from build123d import *

# Parameters (mm, degrees)
SKETCH_1_W          = 30
SKETCH_1_H          = 13
EXTRUDE_1_DEPTH     = 10
SKETCH_2_W          = 24
SKETCH_2_H          = 10
CUT_EXTRUDE_1_DEPTH = 20
SKETCH_3_R          = 3
EXTRUDE_2_DEPTH     = 5
SKETCH_4_R          = 3
CUT_EXTRUDE_2_DEPTH = 39.288379438
FILLET_1_R          = 6


with BuildPart() as part:
    # 草图1 → 凸台-拉伸1 (new, symmetric)
    with BuildSketch(Plane(origin=(0, 0, 0), x_dir=(1, 0, 0), z_dir=(0, 1, 0))):
        Rectangle(SKETCH_1_W, SKETCH_1_H)
    extrude(amount=EXTRUDE_1_DEPTH, both=True)

    # 草图2 → 切除-拉伸1 (cut)
    with BuildSketch(Plane(origin=(0, 0, -6.5), x_dir=(-1, 0, 0), z_dir=(0, 0, -1))):
        with Locations((15, 0)):
            Rectangle(SKETCH_2_W, SKETCH_2_H)
    extrude(amount=-CUT_EXTRUDE_1_DEPTH, mode=Mode.SUBTRACT)

    # 草图3 → 凸台-拉伸2 (add)
    with BuildSketch(Plane(origin=(0, 10, 0), x_dir=(1, 0, 0), z_dir=(0, 1, 0))):
        with BuildLine():
            Line((-3.690899012, 26.00908083), (-15, 6.5))
            Line((-15, 6.5), (-1, 6.5))
            Line((-1, 6.5), (6.712455076, 20.028415898))
            ThreePointArc((6.712455076, 20.028415898), (4.49035189, 28.201710831), (-3.690899012, 26.00908083))
        make_face()
        with Locations(Location((1.5, 23, 0), (0, 0, 270))):
            Circle(SKETCH_3_R, mode=Mode.SUBTRACT)
    extrude(amount=-EXTRUDE_2_DEPTH)

    # 草图4 → 切除-拉伸2 (cut, through all)
    with BuildSketch(Plane(origin=(0, 10, 0), x_dir=(1, 0, 0), z_dir=(0, 1, 0))):
        with Locations(Location((-9, 0, 0), (0, 0, 270))):
            Circle(SKETCH_4_R)
    extrude(amount=-CUT_EXTRUDE_2_DEPTH, mode=Mode.SUBTRACT)

    # 圆角1
    fillet_1_edges = [part.edges().sort_by_distance(p)[0] for p in [
        (-15, -7.5, 6.5),
        (-15, -7.5, -6.5),
        (-15, 7.5, 6.5),
    ]]
    fillet(fillet_1_edges, radius=FILLET_1_R)


solid = part.part
Geometry: final body of the model. Coordinates: model frame, mm. A direction names the side the tool comes from. Coordinates: 2 decimals unless noted, no trailing zeros. Order: outer loops, then holes, each group sorted by start corner. A loop starts at its lowest first (then second) coordinate and runs counter-clockwise, first axis right, second up.
(1) Draft query along Y for faces 5 (the face through (-9.266, 7.535, -16.391)), 6 (the face through (-4, 10, -8)), 7 (the face through (-6, -5, -2)), 8 (the face through (-3, 0, 0)). Return one class per face: pulls with the +Y half, pulls with the -Y half, needs draft (parallel to the pull), parting line crosses it, or undercut.
(2) Section query D-D (y = -8.5). Return the cut outline in (x, z).
(3) Section query A-A (z = 0). Return the cut outline in (x, y).
(4) Section query C-C (z = -23). Return the cut outline in (x, y), plus the area to 3 significant figures.
(5) Access query for faces 1 (the face through (-13.289, 7.535, 4.696)), 2 (the face through (-13.196, -7.535, -4.789)), 3 (the face through (-4, 5, -11)), 4 (the face through (2.802, 7.535, -13.17)). Directions: +Z, -Z, +X, -X, +Y, -Y. A direction counts if a zero-diameter tool reaches every point of the face in a straight line with its end or side. Return the directions, or none.
(6) Section query B-B (x = -0.5). Return the cut outline in (y, z).
(7) Material intervals for probe 1 along X at (y, z) = (-9, 0); probe 2 along Y at (x, z) = (-6, -5); probe 3 along Y at (x, z) = (4, -17.5), sorted ascending.
(8) First-contact query: pin 1 (6 mm diameter, centred on x = -11, y = -7.5, fed in from -Z); pin 2 (3 mm diameter, centred on y = -2.5, z = 0, fed in from -X); pin 3 (7 mm diameter, centred on x = 1.5, z = -23, fed in from -Y). Flat tips, straight axial feed; report the tip coordinate or a pass-through.
Solution:
1. face 5: needs draft
1. face 6: pulls with the +Y half
1. face 7: undercut
1. face 8: undercut
2. outline: (-15, -0.5) arc R6 ccw to (-9, -6.5) - (15, -6.5) - (15, 6.5) - (-9, 6.5) arc R6 ccw to (-15, 0.5) - close; hole circle Ø6 at (-9, 0)
3. outline: (-15, -10) - (-12, -10) - (-12, -5) - (-15, -5) - close; (-15, 5) - (-12, 5) - (-12, 10) - (-15, 10) - close; (-6, -10) - (15, -10) - (15, 10) - (-6, 10) - (-6, 5) - (-3, 5) - (-3, -5) - (-6, -5) - close
4. outline: (-5.44, 5) - (-1.5, 5) - (-1.5, 10) - (-5.44, 10) - close; (4.5, 5) - (7.5, 5) - (7.5, 10) - (4.5, 10) - close
4. area: 34.7 mm2
5. face 1: +Z, -X, +Y, -Y
5. face 2: -Z, -X, -Y
5. face 3: -Z, -X
5. face 4: +X, +Y, -Y
6. outline: (-10, -6.5) - (10, -6.5) - (10, 6.5) - (-10, 6.5) - close; (5, -28.66) - (10, -28.66) - (10, -25.24) - (5, -25.24) - close; (5, -20.76) - (10, -20.76) - (10, -7.38) - (5, -7.38) - close
7. probe 1: x = -15 to -12, -6 to 15
7. probe 2: y = -10 to -5, 5 to 10
7. probe 3: y = 5 to 10
8. pin 1: stops at z = -6.5
8. pin 2: stops at x = -3
8. pin 3: stops at y = 5
